```python
from build123d import *

# Parameters (mm, degrees)
F0_W      = 72
F0_H      = 145
F1_DEPTH  = 90
F2_W      = 109
F2_H      = 65
F3_DEPTH  = 72
F4_W      = 50
F4_H      = 72
F5_DEPTH  = 6
F7_DEPTH  = 25
F8_R      = 12
F9_DEPTH  = 12
F10_DEPTH = 36


with BuildPart() as f1:
    # F0 (on Top) → F1 (new body)
    with BuildSketch(Plane.XY):
        with Locations((4.297932, 22.416884)):
            Rectangle(F0_W, F0_H)
    extrude(amount=F1_DEPTH)

    # F2 (on face) → F3 (cut)
    with BuildSketch(Plane.YZ.offset(40.297932)):
        with Locations((40.416884, 57.5)):
            Rectangle(F2_W, F2_H)
    extrude(amount=-F3_DEPTH, mode=Mode.SUBTRACT)

    # F4 (on face) → F5 (cut)
    with BuildSketch(Plane(origin=(0, 0, 0), x_dir=(1, 0, 0), z_dir=(0, 0, -1))):
        with Locations((15.297932, 14.083116)):
            Rectangle(F4_W, F4_H)
    extrude(amount=-F5_DEPTH, mode=Mode.SUBTRACT)

    # F6 (on face) → F7 (cut)
    with BuildSketch(Plane.XY.offset(25)):
        with BuildLine():
            Line((16.297932, 94.916884), (-7.702068, 94.916884))
            Line((-7.702068, 94.916884), (-7.702068, 44.916884))
            ThreePointArc((-7.702068, 44.916884), (4.297932, 32.916884), (16.297932, 44.916884))
            Line((16.297932, 44.916884), (16.297932, 94.916884))
        make_face()
    extrude(amount=-F7_DEPTH, mode=Mode.SUBTRACT)

    # F8 (on face) → F9 (cut)
    with BuildSketch(Plane.XZ.offset(50.083116)):
        with BuildLine():
            Line((-19.702068, 66), (-31.702068, 66))
            Line((-31.702068, 66), (-31.702068, 30))
            Line((-31.702068, 30), (-19.702068, 30))
            ThreePointArc((-19.702068, 30), (4.297932, 18), (28.297932, 30))
            Line((28.297932, 30), (40.297932, 30))
            Line((40.297932, 30), (40.297932, 66))
            Line((40.297932, 66), (28.297932, 66))
            ThreePointArc((28.297932, 66), (4.297932, 78), (-19.702068, 66))
        make_face()
        with Locations((4.297932, 48)):
            Circle(F8_R, mode=Mode.SUBTRACT)
    extrude(amount=-F9_DEPTH, mode=Mode.SUBTRACT)

    # F8 (on face) → F10 (cut)
    with BuildSketch(Plane.XZ.offset(50.083116)):
        with Locations((4.297932, 48)):
            Circle(F8_R)
    extrude(amount=-F10_DEPTH, mode=Mode.SUBTRACT)


solid = f1.part
```
Check sheet for the modelled part. Datum: model origin and axes. Units: mm. A direction names the side the tool comes from. Coordinates: 2 decimals unless noted, no trailing zeros. Loops run counter-clockwise (first coordinate to the right, second up) from the corner with the lowest first, then second, coordinate; pieces in that order, holes last.
1) Material ranges on probe 1 along Z at (x, y) = (-29, 62); probe 2 along Y at (x, z) = (-25, 26); probe 3 along X at (y, z) = (-21.5, 37), recorded low to high.
2) Sectioned sample at D-D (z = 23.5). Record the boundary of the cut face in (x, y).
3) Gauge pin test, flat ends, axial feed: pin 1 (6 mm diameter, centred on x = 15.5, y = 70.5, fed in from +Z); pin 2 (8 mm diameter, centred on x = 27.5, z = 56, fed in from +Y); pin 3 (25 mm diameter, centred on x = 5.5, y = 2.5, fed in from -Z); pin 4 (6 mm diameter, centred on x = 12.5, z = 46, fed in from +Y). Record the tip position at first contact, or that the pin passes through.
4) Sectioned sample at C-C (y = -12). Record the boundary of the cut face in (x, z).
5) Sectioned sample at B-B (z = 48). Record the boundary of the cut face in (x, y).
6) Access from +Z, -Z, +X, -X, +Y, -Y to the whole of each face (thin tool, end or side, straight path). Record for faces 1 (the face through (4.687, -44.167, 77.997)), 2 (the face through (-7.702, 70, 13)), 3 (the face through (-26, -44, 66)).
7) Sectioned sample at A-A (y = 80.5). Record the boundary of the cut face in (x, z), and give its area (3 significant figures).
Check sheet entries:
1. probe 1: z = 0 to 25
1. probe 2: y = -50.08 to -14.08
1. probe 3: x = -31.7 to -0.5, 9.09 to 40.3
2. outline: (-31.7, -50.08) - (-13.02, -50.08) - (-13.02, -38.08) - (21.61, -38.08) - (21.61, -50.08) - (40.3, -50.08) - (40.3, 94.92) - (16.3, 94.92) - (16.3, 44.92) arc R12 cw to (-7.7, 44.92) - (-7.7, 94.92) - (-31.7, 94.92) - close
3. pin 1: stops at z = 25
3. pin 2: stops at y = -14.08
3. pin 3: stops at z = 6
3. pin 4: passes through
4. outline: (-31.7, 0) - (-9.7, 0) - (-9.7, 6) - (40.3, 6) - (40.3, 25) - (-31.7, 25) - close
5. outline: (-31.7, -38.08) - (-7.7, -38.08) - (-7.7, -14.08) - (-31.7, -14.08) - close; (16.3, -38.08) - (40.3, -38.08) - (40.3, -14.08) - (16.3, -14.08) - close
6. face 1: -Y
6. face 2: +Z, -Z, +Y
6. face 3: +X, -X, -Y
7. outline: (-31.7, 0) - (-7.7, 0) - (-7.7, 25) - (-31.7, 25) - close; (16.3, 0) - (40.3, 0) - (40.3, 25) - (16.3, 25) - close
7. area: 1,200 mm2
